Autodesk Inventor part; units mm, degrees
ref_plane "YZ Plane" through (0, 0, 0) normal (1, 0, 0) x (0, 1, 0)
ref_plane "XZ Plane" through (0, 0, 0) normal (0, 1, 0) x (-1, 0, 0)
ref_plane "XY Plane" through (0, 0, 0) normal (0, 0, 1) x (1, 0, 0)
sketch "Sketch1" plane through (0, 0, 0) normal (1, 0, 0) x (0, 1, 0)
  point P0 (0, 0)
sketch "Sketch2" plane through (0, 0, 0) normal (0, 0, 1) x (1, 0, 0)
  line L0 (0, 0) -> (500, 0)
  line L1 (650, -710) -> (500, 0)
  line L2 (-150, -710) -> (0, 0)
  line L3 (-22.2287, -226.1612) -> (20.2701, -25)
  line L4 (-22.2287, -226.1612) -> (-124.4482, -710)
  line L5 (572.0133, -461.8084) -> (479.7299, -25)
  line L6 (572.0133, -461.8084) -> (624.4482, -710)
  line L7 (20.2701, -25) -> (479.7299, -25)
  line L8 (-150, -710) -> (-124.4482, -710)
  line L9 (624.4482, -710) -> (650, -710)
  dimension "d0" = 500
sketch "Sketch3" plane through (0, 0, 0) normal (0, 0, 1) x (1, 0, 0)
  point P0 (0, 0)
extrude "Extrusion1" add sketch "Sketch2" along normal blind 70
properties part number "leg" material "Steel, Galvanized"
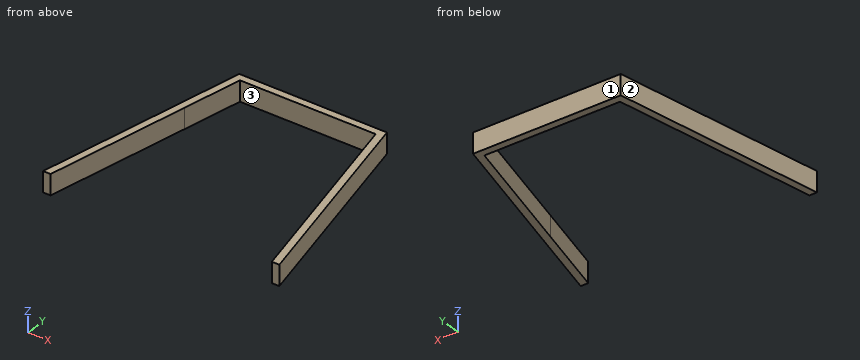
Check sheet for the modelled part. Datum: model origin and axes. Units: mm. Face numbers are marked on the shaded views. Give positions to 0.01 mm unless a question says otherwise; leave off trailing zeros. Loops run counter-clockwise (first coordinate to the right, second up) from the corner with the lowest first, then second, coordinate; pieces in that order, holes last. Notation, with made-up numbers: M 6.25,-38 L 21.25,-38 A20 ccw 21.25,-30 Z; hole C -14.5,-3.75 d10. An arc over 180 degrees is marked long. Use a Markdown table: item, result. Add a question column.
Q1. Sectioned sample at A-A, the plane z = 52. Record the cut outline in (x, y).
Q2. Scan lines: line 1 along Y through (x, z) = (56.5, 43); line 2 along X through (y, z) = (-216, 63.5); line 3 along X through (y, z) = (-444, 15.5). Record each from-to range of solid material in increasing order. Write a range as [from, to].
Q3. Sectioned sample at B-B, the plane y = -501.5. Record the cut outline in (x, z).
Q4. Sectioned sample at C-C, the plane x = 42.5. Record the cut outline in (y, z), then the cut area to 3 significant figures.
Q5. Mould release check, pull along X, two halves, no side actions. Record for the marked faces 1, 2 and 3: pulls with the +X half, pulls with the -X half, needs draft (parallel to the pull), parting line crosses it, or undercut.
Q6. Sectioned sample at D-D, the plane y = -368. Record the cut outline in (x, z), then the cut area to 3 significant figures.
Q7. Go/stop test with flat-tipped pins: pin 1 (3 mm diameter, centred on y = -621, z = 49.5, fed in from -X); pin 2 (21 mm diameter, centred on x = 274, z = 27, fed in from -Y); pin 3 (1.5 mm diameter, centred on y = -425, z = 17.5, fed in from +X). Record where each tip stops, or that it passes through.
Verdict:
| question | item | result |
|---|---|---|
| 1 | outline | M -150,-710 L -124.45,-710 L -22.23,-226.16 L 20.27,-25 L 479.73,-25 L 572.01,-461.81 L 624.45,-710 L 650,-710 L 500,0 L 0,0 Z |
| 2 | line 1 | [-25, 0] |
| 2 | line 2 | [-45.63, -20.08], [520.08, 545.63] |
| 2 | line 3 | [-93.8, -68.25], [568.25, 593.8] |
| 3 | outline | M -105.95,0 L -80.4,0 L -80.4,70 L -105.95,70 Z; M 580.4,0 L 605.95,0 L 605.95,70 L 580.4,70 Z |
| 4 | outline | M -25,0 L 0,0 L 0,70 L -25,70 Z |
| 4 | area | 1,750 mm^2 |
| 5 | face 1 | needs draft |
| 5 | face 2 | pulls with the -X half |
| 5 | face 3 | undercut |
| 6 | outline | M -77.75,0 L -52.19,0 L -52.19,70 L -77.75,70 Z; M 552.19,0 L 577.75,0 L 577.75,70 L 552.19,70 Z |
| 6 | area | 3,580 mm^2 |
| 7 | pin 1 | x = -131.51 |
| 7 | pin 2 | y = -25 |
| 7 | pin 3 | x = 589.95 |
